from build123d import *

# Parameters (mm, degrees)
F1_DEPTH = 2.54
F2_W     = 10.16
F2_H     = 10.16
F3_DEPTH = 2.54
F5_DEPTH = 2.54
F6_W     = 25.4
F6_H     = 2.794
F7_DEPTH = 25.4


with BuildPart() as f1:
    # F0 (on Top) → F1 (new body)
    with BuildSketch(Plane.XY):
        with BuildLine():
            Line((206.375, -73.81875), (206.375, 73.81875))
            ThreePointArc((206.375, 73.81875), (196.145704, 98.514454), (171.45, 108.74375))
            Line((171.45, 108.74375), (-171.45, 108.74375))
            ThreePointArc((-171.45, 108.74375), (-196.145704, 98.514454), (-206.375, 73.81875))
            Line((-206.375, 73.81875), (-206.375, -73.81875))
            ThreePointArc((-206.375, -73.81875), (-196.145704, -98.514454), (-171.45, -108.74375))
            Line((-171.45, -108.74375), (171.45, -108.74375))
            ThreePointArc((171.45, -108.74375), (196.145704, -98.514454), (206.375, -73.81875))
        make_face()
        with BuildLine():
            ThreePointArc((187.325, -73.81875), (182.67532, -85.04407), (171.45, -89.69375))
            Line((171.45, -89.69375), (-171.45, -89.69375))
            ThreePointArc((-171.45, -89.69375), (-182.67532, -85.04407), (-187.325, -73.81875))
            Line((-187.325, -73.81875), (-187.325, 73.81875))
            ThreePointArc((-187.325, 73.81875), (-182.67532, 85.04407), (-171.45, 89.69375))
            Line((-171.45, 89.69375), (171.45, 89.69375))
            ThreePointArc((171.45, 89.69375), (182.67532, 85.04407), (187.325, 73.81875))
            Line((187.325, 73.81875), (187.325, -73.81875))
        make_face(mode=Mode.SUBTRACT)
    extrude(amount=F1_DEPTH)

    # F2 (on face) → F3 (cut, through all)
    with BuildSketch(Plane.XY.offset(2.54)):
        with Locations((-131.445, 94.77375)):
            Rectangle(F2_W, F2_H)
        with Locations((114.6175, 94.77375)):
            Rectangle(F2_W, F2_H)
    extrude(amount=-F3_DEPTH, mode=Mode.SUBTRACT)

    # F4 (on face) → F5 (join, through all)
    with BuildSketch(Plane.XY.offset(2.54)):
        with BuildLine():
            ThreePointArc((-186.176704, 79.746635), (-178.185192, 80.553942), (-177.377885, 88.545454))
            ThreePointArc((-177.377885, 88.545454), (-182.67532, 85.04407), (-186.176704, 79.746635))
        make_face()
        with BuildLine():
            ThreePointArc((186.176704, 79.746635), (182.67532, 85.04407), (177.377885, 88.545454))
            ThreePointArc((177.377885, 88.545454), (178.185192, 80.553942), (186.176704, 79.746635))
        make_face()
        with BuildLine():
            ThreePointArc((186.176704, -79.746635), (178.185192, -80.553942), (177.377885, -88.545454))
            ThreePointArc((177.377885, -88.545454), (182.67532, -85.04407), (186.176704, -79.746635))
        make_face()
        with BuildLine():
            ThreePointArc((-177.377885, -88.545454), (-178.185192, -80.553942), (-186.176704, -79.746635))
            ThreePointArc((-186.176704, -79.746635), (-182.67532, -85.04407), (-177.377885, -88.545454))
        make_face()
    extrude(amount=-F5_DEPTH)

    # F6 (on face) → F7 (cut)
    with BuildSketch(Plane.XY.offset(2.54)):
        with Locations((-107.315, 94.77375)):
            Rectangle(F6_W, F6_H)
        with Locations((138.7475, 94.77375)):
            Rectangle(F6_W, F6_H)
    extrude(amount=-F7_DEPTH, mode=Mode.SUBTRACT)


solid = f1.part
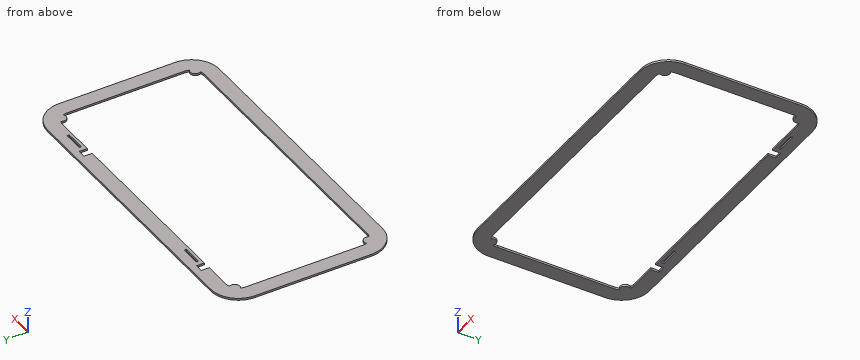
Verification items for the finished model (mm, model axes). Round coordinates to 2 decimals unless told otherwise and drop trailing zeros. Loops run counter-clockwise (first coordinate to the right, second up) from the corner with the lowest first, then second, coordinate; pieces in that order, holes last. Notation, with made-up numbers: (26.5, -15.5) - (62.5, -15.5) arc R28 ccw to (62.5, 22.5) - close; hole circle Ø10 at (60, 53). An arc over 180 degrees is marked (long way). Answer in a Markdown table with one row per item. Add a question column.
Q1. Section check B-B on y = -28.5. Enter the section's corners in (x, z) (3 decimals).
Q2. Section check C-C on z = 1.9. State how many separate pieces and enclosed holes the cut face has, plus the area to 3 significant figures.
Q3. Section check A-A on x = -28.5. Enter the section's corners in (y, z).
Q4. Gauge pin test, flat ends, axial feed: pin 1 (1.5 mm diameter, centred on y = 82.5, z = 1, fed in from -X); pin 2 (1.3 mm diameter, centred on y = 94.5, z = 1.5, fed in from +X); pin 3 (1.3 mm diameter, centred on y = 97, z = 1.5, fed in from -X). Record the tip position at first contact, or that the pin passes through.
Q5. Material ranges on line 1 (Y direction, x = 143, z = 0.85); line 2 (X direction, y = -25, z = 0.4) (3 decimals); line 3 (Y direction, x = 13, z = 0.5), recorded low to high.
Found:
| question | item | result |
|---|---|---|
| 1 | outline | (-206.375, 0) - (-187.325, 0) - (-187.325, 2.54) - (-206.375, 2.54) - close; (187.325, 0) - (206.375, 0) - (206.375, 2.54) - (187.325, 2.54) - close |
| 2 | separate pieces | 1 |
| 2 | enclosed holes | 3 |
| 2 | area | 21,600 mm² |
| 3 | outline | (-108.74, 0) - (-89.69, 0) - (-89.69, 2.54) - (-108.74, 2.54) - close; (89.69, 0) - (108.74, 0) - (108.74, 2.54) - (89.69, 2.54) - close |
| 4 | pin 1 | stops at x = -205.46 |
| 4 | pin 2 | stops at x = 200.06 |
| 4 | pin 3 | stops at x = -198.14 |
| 5 | line 1 | y = -108.74 to -89.69, 89.69 to 93.38, 96.17 to 108.74 |
| 5 | line 2 | x = -206.375 to -187.325, 187.325 to 206.375 |
| 5 | line 3 | y = -108.74 to -89.69, 89.69 to 108.74 |
